CAD build for the part. Positions are in the model's coordinates, mm. A direction names the side the tool comes from. Coordinates: 2 decimals unless noted, no trailing zeros. Loops run counter-clockwise (first coordinate to the right, second up) from the corner with the lowest first, then second, coordinate; pieces in that order, holes last. Notation, with made-up numbers: (71, -27.5) -> (82, -27.5) arc R26 ccw to (82, -5.5) -> close; hole circle Ø8 at (-30.5, -11). An arc over 180 degrees is marked (long way). Write item = value, one per line. Start each with the question number.
(1) Band-saw the part on D-D (x = 825.5). Write the cut outline in (y, z), and give its area (3 significant figures).
(2) Band-saw the part on C-C (x = 165). Write the cut outline in (y, z), and give its area (3 significant figures).
(3) Drill centre lines: line 1 (X direction, y = -4.5, z = -49); line 2 (X direction, y = -6.75, z = -189); line 3 (Z direction, x = 159, y = -7.75). Where is each one in solid material? Low to high. Write a range as from..to.
(4) Flat gauge pins, fed straight in: P1, Ø5, axis at x = 554, y = -14.5, coming from the -Z side; P2, Ø5.5, axis at x = -241, y = -10, coming from the -Z side; P3, Ø1, axis at y = -7, z = 144, coming from the -X side. Where does each tip first touch, or does it go through?
(5) Band-saw the part on A-A (z = -144). Write the cut outline in (x, y).
(6) Band-saw the part on B-B (z = 17). Write the cut outline in (x, y).
(7) Pull direction X, two halves, no side cores. Call faces 3 (the face through (1510.17, -8.87, 345.79)), 4 (the face through (-155.266, -8.874, 230.057)), 5 (the face through (621, -18, 255)): +X half, -X half, draft (parallel to the pull), parting line (faces both ways), or undercut.
(8) Tool access for faces 1 (the face through (1404.73, -8.87, 230.62)), 2 (the face through (-259.736, -8.874, 346.338)): list every direction of +Z, -Z, +X, -X, +Y, -Y with a clear straight run to the whole face (end or side of a thin tool).
```python
from build123d import *

# Parameters (mm, degrees)
F1_DEPTH = 18


# Not quite as in the source:
# - ends of sketch curves that miss each other by under 0.0002 mm in the source are joined


with BuildPart() as f1:
    # F0 (on Front) → F1 (new body)
    with BuildSketch(Plane.XZ):
        with BuildLine():
            Line((1444.9999982887, 361), (1444.9999982887, 379))
            Line((1444.9999982887, 379), (1418.9999982887, 379))
            Line((1418.9999982887, 379), (1418.9999982887, 361.0032042947))
            Line((1418.9999982887, 361.0032042947), (1418.9999982887, 361))
            ThreePointArc((1418.9999982887, 361), (1414.9978620926, 357.0032048651), (1410.9999984313, 361.0042723931))
            Line((1410.9999984313, 361.0042723931), (918.9999984313, 361.0042723931))
            ThreePointArc((918.9999984313, 361.0042723931), (914.9999984313, 357.0042723931), (910.9999984313, 361.0042723931))
            Line((910.9999984313, 361.0042723931), (910.9999984313, 379.0042723931))
            Line((910.9999984313, 379.0042723931), (884.9999984313, 379.0042723931))
            Line((884.9999984313, 379.0042723931), (884.9999984313, 361.0055952483))
            Line((884.9999984313, 361.0055952483), (884.9999984313, 361.0042723931))
            ThreePointArc((884.9999984313, 361.0042723931), (880.9986755762, 357.005595467), (876.9999986501, 361.0069181034))
            Line((876.9999986501, 361.0069181034), (372.9999978512, 361.1735978616))
            ThreePointArc((372.9999978512, 361.1735978616), (368.9986752099, 357.1749209454), (364.9999982887, 361.1762435819))
            Line((364.9999982887, 361.1762435819), (364.9999982887, 379.1762435819))
            Line((364.9999982887, 379.1762435819), (338.9999982887, 379.1762435819))
            Line((338.9999982887, 379.1762435819), (338.9999982887, 361.1783797782))
            ThreePointArc((338.9999982887, 361.1783797782), (334.9999982887, 357.1783797782), (330.9999982887, 361.1783797782))
            Line((330.9999982887, 361.1783797782), (-161.0000017113, 361.1783797782))
            ThreePointArc((-161.0000017113, 361.1783797782), (-165.0000017113, 357.1783797782), (-169.0000017113, 361.1783797782))
            Line((-169.0000017113, 361.1783797782), (-169.0000017113, 379.1783797782))
            Line((-169.0000017113, 379.1783797782), (-195.0000017113, 379.1783797782))
            Line((-195.0000017113, 379.1783797782), (-195.0000012844, 361.180516095))
            ThreePointArc((-195.0000012844, 361.180516095), (-198.9999999526, 357.1805172846), (-202.9999987156, 361.1805160001))
            Line((-202.9999987156, 361.1805160001), (-215.9862284595, 361.1805160001))
            Line((-215.9862284595, 361.1805160001), (-233.9862284595, 361.1805160001))
            Line((-233.9862284595, 361.1805160001), (-244.90749278, 361.1805160001))
            Line((-244.90749278, 361.1805160001), (-274.9862284595, 331.0746893941))
            Line((-274.9862284595, 331.0746893941), (-254.9862284595, -376.2833213137))
            Line((-254.9862284595, -376.2833213137), (-233.9862284595, -376.2833213137))
            Line((-233.9862284595, -376.2833213137), (-233.9862284595, -16.2833213137))
            ThreePointArc((-233.9862284595, -16.2833213137), (-237.9862284595, -12.2833213137), (-233.9862284595, -8.2833213137))
            Line((-233.9862284595, -8.2833213137), (-215.9862284595, -8.2833213137))
            ThreePointArc((-215.9862284595, -8.2833213137), (-211.9862284595, -12.2833213137), (-215.9862284595, -16.2833213137))
            Line((-215.9862284595, -16.2833213137), (-215.9862284595, -376.2833213137))
            Line((-215.9862284595, -376.2833213137), (-194.9862284595, -376.2833213137))
            Line((-194.9862284595, -376.2833213137), (-174.9862284595, 210.3365797868))
            Line((-174.9862284595, 210.3365797868), (-134.9862284595, 250.3365797868))
            Line((-134.9862284595, 250.3365797868), (1385.0137715405, 250.3365797868))
            Line((1385.0137715405, 250.3365797868), (1425.0137715405, 210.3365797868))
            Line((1425.0137715405, 210.3365797868), (1445.0137715405, -376.2833213137))
            Line((1445.0137715405, -376.2833213137), (1466.022162316, -375.6897371419))
            Line((1466.022162316, -375.6897371419), (1466.022162316, -15.6897371419))
            ThreePointArc((1466.022162316, -15.6897371419), (1462.0221624552, -11.6907923518), (1466.0200518963, -7.6897376986))
            Line((1466.0200518963, -7.6897376986), (1466.022162316, -7.6897371419))
            Line((1466.022162316, -7.6897371419), (1484.020051896, -7.6897371419))
            ThreePointArc((1484.020051896, -7.6897371419), (1488.020051896, -11.6897371419), (1484.020051896, -15.6897371419))
            Line((1484.020051896, -15.6897371419), (1484.020051896, -375.7643703854))
            Line((1484.020051896, -375.7643703854), (1505.0116611204, -376.3579545571))
            Line((1505.0116611204, -376.3579545571), (1525.0137715405, 331))
            Line((1525.0137715405, 331), (1494.9069982887, 361))
            Line((1494.9069982887, 361), (1466.022162316, 361))
            Line((1466.022162316, 361), (1452.9999982887, 361))
            ThreePointArc((1452.9999982887, 361), (1448.9999982887, 357), (1444.9999982887, 361))
        make_face()
    extrude(amount=F1_DEPTH)


solid = f1.part
```
Findings below:
q1.outline = (-18, 250.34) -> (0, 250.34) -> (0, 361.02) -> (-18, 361.02) -> close
q1.area = 1,990 mm²
q2.outline = (-18, 250.34) -> (0, 250.34) -> (0, 361.18) -> (-18, 361.18) -> close
q2.area = 2,000 mm²
q3.line_1 = -264.24..-233.99, -215.99..-183.83, 1433.86..1466.02, 1484.02..1514.27
q3.line_2 = -260.28..-233.99, -215.99..-188.6, 1438.63..1466.02, 1484.02..1510.31
q3.line_3 = 250.34..361.18
q4.P1 = 250.34
q4.P2 = -376.28
q4.P3 = -269.71
q5.outline = (-261.55, -18) -> (-233.99, -18) -> (-233.99, 0) -> (-261.55, 0) -> close; (-215.99, -18) -> (-187.07, -18) -> (-187.07, 0) -> (-215.99, 0) -> close; (1437.09, -18) -> (1466.02, -18) -> (1466.02, 0) -> (1437.09, 0) -> close; (1484.02, -18) -> (1511.58, -18) -> (1511.58, 0) -> (1484.02, 0) -> close
q6.outline = (-266.11, -18) -> (-181.58, -18) -> (-181.58, 0) -> (-266.11, 0) -> close; (1431.61, -18) -> (1516.13, -18) -> (1516.13, 0) -> (1431.61, 0) -> close
q7.face_3 = +X half
q7.face_4 = undercut
q7.face_5 = draft
q8.face_1 = -Z, +Y, -Y
q8.face_2 = +Z, -X, +Y, -Y
